```python
from build123d import *

# Parameters (mm, degrees)
SKETCH_W        = 70
SKETCH_H        = 30
PAD_DEPTH       = 5.5
SKETCH001_W     = 114.652
SKETCH001_H     = 7
POCKET_DEPTH    = 24
PAD001_DEPTH    = 25
SKETCH004_R     = 12.8
POCKET001_DEPTH = 30.174648


with BuildPart() as part:
    # Sketch → Pad (new body, symmetric)
    with BuildSketch(Plane.XY):
        with Locations((-35, -15)):
            Rectangle(SKETCH_W, SKETCH_H)
    extrude(amount=PAD_DEPTH, both=True)

    # Sketch001 → Pocket (cut)
    with BuildSketch(Plane.XZ.offset(30)):
        with Locations((-38.5063, 0)):
            Rectangle(SKETCH001_W, SKETCH001_H)
    extrude(amount=-POCKET_DEPTH, mode=Mode.SUBTRACT)

    # Sketch003 → Pad001 (new body)
    with BuildSketch(Plane(origin=(0, 0, -5.5), x_dir=(1, 0, 0), z_dir=(0, 0, -1))):
        Polygon((-38.644903, 0), (-1, 0), (1.923717, 9.563048), (-32.503254, 20.088429), align=None)
        Polygon((-38.644903, 0), (-1, 0), align=None)
    extrude(amount=PAD001_DEPTH)

    # Sketch004 → Pocket001 (cut, through all)
    with BuildSketch(Plane(origin=(2.838236, -9.283451, 0), x_dir=(0.956305, 0.292372, 0), z_dir=(0.292372, -0.956305, 0))):
        with Locations((-18.956305, -30.5)):
            Circle(SKETCH004_R)
    extrude(amount=-POCKET001_DEPTH, mode=Mode.SUBTRACT)


solid = part.part
```
Model file for the job. Use its own axes, mm. A direction names the side the tool comes from. Give positions to 0.01 mm unless a question says otherwise; leave off trailing zeros. Loops run counter-clockwise (first coordinate to the right, second up) from the corner with the lowest first, then second, coordinate; pieces in that order, holes last. Notation, with made-up numbers: (62.25, -25.5) - (110.25, -25.5) arc R21 cw to (110.25, -19.5) - close; hole circle Ø5 at (61.5, 52.25). An arc over 180 degrees is marked (long way). One line per item, written item: value. Start each with the question number.
1. Slice it at C-C (x = -65). List the corners of the cut face in (y, z), plus the area to 3 significant figures.
2. Slice it at A-A (y = -21). List the corners of the cut face in (x, z).
3. Which spindle directions (+Z, -Z, +X, -X, +Y, -Y) get a long thin tool onto all of the face, cutting with end or side? Do faces 1 (the flat face through (0, -12, 4)), 2 (the flat face through (-15.049, -14.752, -15.047)), 3 (the flat face through (-35.531, -10.185, -17.825)), 4 (the flat face through (0.44, -4.71, -17.82)), 5 (the flat face through (-35, -18, 3.5)). Say none if no direction does.
4. Slice it at B-B (z = -21.5). List the corners of the cut face in (x, y).
5. Slice it at D-D (z = -2.5). List the corners of the cut face in (x, y).
6. Probe L1, parallel to Z at x = -31.5, y = -25.5; L2, parallel to Z at x = -33, y = -7; L3, parallel to Y at x = -37, z = -2.5. List the from-to ranges inside material, lowest first. Write a range as from..to.
7. Pin check, flat tips, straight feed: pin 1 (7 mm diameter, centred on x = -51, y = -17, fed in from -Z); pin 2 (3 mm diameter, centred on x = -13.5, y = -15.5, fed in from -Z); pin 3 (3.5 mm diameter, centred on y = -16, z = 2, fed in from +X). Stop position of each tip, or through.
Solution:
1. outline: (-30, -5.5) - (0, -5.5) - (0, 5.5) - (-30, 5.5) - (-30, 3.5) - (-6, 3.5) - (-6, -3.5) - (-30, -3.5) - close
1. area: 162 mm^2
2. outline: (-70, -5.5) - (0, -5.5) - (0, -3.5) - (-70, -3.5) - close; (-70, 3.5) - (0, 3.5) - (0, 5.5) - (-70, 5.5) - close
3. face 1: +Z, +X, +Y, -Y
3. face 2: -Z, +X, -Y
3. face 3: -Z, -X, -Y
3. face 4: -Z, +X, +Y
3. face 5: +X, -X, -Y
4. outline: (-38.64, 0) - (-32.5, -20.09) - (-23.99, -17.49) - (-29.34, 0) - close; (-10.3, 0) - (-6.59, -12.16) - (1.92, -9.56) - (-1, 0) - close
5. outline: (-70, -6) - (0, -6) - (0, 0) - (-70, 0) - close
6. L1: z = -5.5..-3.5, 3.5..5.5
6. L2: z = -30.5..-3.5, 3.5..5.5
6. L3: y = -6..0
7. pin 1: stops at z = -5.5
7. pin 2: stops at z = -17.94
7. pin 3: stops at x = 0
